```python
from build123d import *

# Parameters (mm, degrees)
BOSS_EXTRUDE1_DEPTH = 76.2


with BuildPart() as part:
    # Sketch1 → Boss-Extrude1 (new body)
    with BuildSketch(Plane(origin=(0, 0, 0), x_dir=(1, 0, 0), z_dir=(0, 1, 0))):
        with BuildLine():
            Line((-257.175, 0), (257.175, 0))
            Line((257.175, 0), (257.175, 5.4))
            ThreePointArc((257.175, 5.4), (236.438160108, 55.463160108), (186.375, 76.2))
            Line((186.375, 76.2), (-186.375, 76.2))
            ThreePointArc((-186.375, 76.2), (-236.438160108, 55.463160108), (-257.175, 5.4))
            Line((-257.175, 5.4), (-257.175, 0))
        make_face()
        with BuildLine():
            Line((254.635, 5.4), (254.635, 2.54))
            Line((254.635, 2.54), (-254.635, 2.54))
            Line((-254.635, 2.54), (-254.635, 5.4))
            ThreePointArc((-254.635, 5.4), (-234.642108884, 53.667108884), (-186.375, 73.66))
            Line((-186.375, 73.66), (186.375, 73.66))
            ThreePointArc((186.375, 73.66), (234.642108884, 53.667108884), (254.635, 5.4))
        make_face(mode=Mode.SUBTRACT)
    extrude(amount=BOSS_EXTRUDE1_DEPTH)


solid = part.part
```
Model file for the job. Use its own axes, mm. A direction names the side the tool comes from. Coordinates: 2 decimals unless noted, no trailing zeros. Loops run counter-clockwise (first coordinate to the right, second up) from the corner with the lowest first, then second, coordinate; pieces in that order, holes last. Notation, with made-up numbers: (-32.5, 25.5) - (-8.5, 25.5) arc R17 ccw to (-8.5, 32.5) - close; hole circle Ø10 at (88.5, 75). An arc over 180 degrees is marked (long way). Write item = value, one per line. Start each with the question number.
Item 1: Saw through at B-B, the plane z = -66.5. List the corners of the cut face in (x, y), then the cut area to 3 significant figures.
Item 2: Pull direction Z, two halves, no side cores. Call faces 1 (the face through (-3, 38, -73.66)), 2 (the face through (3, 38, -76.2)), 3 (the face through (-1, 76.2, -2)): +Z half, -Z half, draft (parallel to the pull), parting line (faces both ways), or undercut.
Item 3: Drop a flat-ended pin along its axis: pin 1 Ø12 at (y, z) = (8.5, -49.5) entering from +X. Give the stop position or say it passes through.
Item 4: 3-axis set-ups, long thin cutter, end or side, ignore diameter. For faces 4 (the face through (234.108, 37.567, -54.195)), 5 (the face through (236.986, 37.567, -54.91)): which of +Z, -Z, +X, -X, +Y, -Y reach the whole face in a straight line?
Item 5: Saw through at A-A, the plane x = -153. List the corners of the cut face in (y, z), then the cut area to 3 significant figures.
Item 6: Saw through at C-C, the plane y = 7. List the corners of the cut face in (x, z) (3 decimals), then the cut area to 3 significant figures.
Item 7: Wall check: probe 1 along Z at (x, y) = (-86, 49); probe 2 along X at (y, z) = (54, -5.5); probe 3 along X at (y, z) = (35, -9.5). Give the ranges that are in metal, low to high. Write a range as [from, to].
Answers:
q1.outline = (-222.14, 0) - (-216.81, 0) - (-216.81, 76.2) - (-222.14, 76.2) - close; (216.81, 0) - (222.14, 0) - (222.14, 76.2) - (216.81, 76.2) - close
q1.area = 813 mm2
q2.face_1 = undercut
q2.face_2 = -Z half
q2.face_3 = draft
q3.pin_1 = 246.05
q4.face_4 = +Y, -Y
q4.face_5 = -Z, +X, +Y, -Y
q5.outline = (0, -76.2) - (76.2, -76.2) - (76.2, -73.66) - (0, -73.66) - close; (0, -2.54) - (76.2, -2.54) - (76.2, 0) - (0, 0) - close
q5.area = 387 mm2
q6.outline = (-257.175, -5.4) arc R70.8 ccw to (-186.375, -76.2) - (186.375, -76.2) arc R70.8 ccw to (257.175, -5.4) - (257.175, 0) - (-257.175, 0) - close; hole (-254.635, -5.4) arc R68.26 ccw to (-186.375, -73.66) - (186.375, -73.66) arc R68.26 ccw to (254.635, -5.4) - (254.635, -2.54) - (-254.635, -2.54) - close
q6.area = 2,820 mm2
q7.probe_1 = [-76.2, -73.66], [-2.54, 0]
q7.probe_2 = [-257.17, -254.63], [254.63, 257.17]
q7.probe_3 = [-257.06, -254.51], [254.51, 257.06]
